For this review, take the finished solid that the model builds, in its own axes (mm). A direction names the side the tool comes from. Coordinates: 2 decimals unless noted, no trailing zeros. Loops run counter-clockwise (first coordinate to the right, second up) from the corner with the lowest first, then second, coordinate; pieces in that order, holes last. Notation, with made-up numbers: M -7,70.5 L 8,70.5 A28 cw 8,105.5 Z; hole C 26.25,64.25 d3. An arc over 180 degrees is marked long. Write item = value, one per line.
from build123d import *

# Parameters (mm, degrees)
SKETCH1_W           = 170
SKETCH1_H           = 130
BOSS_EXTRUDE1_DEPTH = 5
SKETCH2_W           = 67
SKETCH2_H           = 85
CUT_EXTRUDE1_DEPTH  = 108.121426428
SKETCH3_W           = 5
SKETCH3_H           = 5.833333
CUT_EXTRUDE2_DEPTH  = 108.121426428
FILLET1_R           = 15


with BuildPart() as part:
    # Sketch1 → Boss-Extrude1 (new body)
    with BuildSketch(Plane(origin=(0, 0, 0), x_dir=(1, 0, 0), z_dir=(0, 1, 0))):
        Rectangle(SKETCH1_W, SKETCH1_H)
    extrude(amount=BOSS_EXTRUDE1_DEPTH)

    # Sketch2 → Cut-Extrude1 (cut, through all)
    with BuildSketch(Plane(origin=(0, 5, 0), x_dir=(1, 0, 0), z_dir=(0, 1, 0))):
        Rectangle(SKETCH2_W, SKETCH2_H)
    extrude(amount=-CUT_EXTRUDE1_DEPTH, mode=Mode.SUBTRACT)

    # Sketch3 → Cut-Extrude2 (cut, through all)
    with BuildSketch(Plane(origin=(0, 5, 0), x_dir=(1, 0, 0), z_dir=(0, 1, 0))):
        with Locations((-36, -33.7500005)):
            Rectangle(SKETCH3_W, SKETCH3_H)
        with Locations((36, 33.7500005)):
            Rectangle(SKETCH3_W, SKETCH3_H)
        with Locations((-36, 33.7500005)):
            Rectangle(SKETCH3_W, SKETCH3_H)
        with Locations((36, -33.7500005)):
            Rectangle(SKETCH3_W, SKETCH3_H)
    extrude(amount=-CUT_EXTRUDE2_DEPTH, mode=Mode.SUBTRACT)

    # Fillet1
    fillet1_edges = [part.edges().sort_by_distance(p)[0] for p in [
        (85, 2.5, 65),
        (-85, 2.5, 65),
        (-85, 2.5, -65),
        (85, 2.5, -65),
    ]]
    fillet(fillet1_edges, radius=FILLET1_R)


solid = part.part
Q1. Machinability: for faces 1 (the face through (33.5, 3, -40)), 2 (the face through (80.49, 2.54, -60.72)), which of the approach directions +Z, -Z, +X, -X, +Y, -Y give a long, thin tool a straight path to every point of the face, cutting with its end or side? Answer none if there is none.
Solved:
face_1 = +Y, -Y
face_2 = -Z, +X, +Y, -Y
Q2. For line 1 along Z through (x, y) = (-35, 1.8); line 2 along X through (y, z) = (1.4, -26.5); line 3 along Z through (x, y) = (8, 2.95), list the stretches that pass through material, from the lowest coordinate up.
Solved:
line_1 = -65 to -36.67, -30.83 to 30.83, 36.67 to 65
line_2 = -85 to -33.5, 33.5 to 85
line_3 = -65 to -42.5, 42.5 to 65
Q3. Add section A-A (x = -17). Write out the cut boundary in (y, z), and give its area (3 significant figures).
Solved:
outline = M 0,-65 L 5,-65 L 5,-42.5 L 0,-42.5 Z; M 0,42.5 L 5,42.5 L 5,65 L 0,65 Z
area = 225 mm²
Q4. Add section B-B (y = 1.2). Write out the cut boundary in (x, z).
Solved:
outline = M -85,-50 A15 ccw -70,-65 L 70,-65 A15 ccw 85,-50 L 85,50 A15 ccw 70,65 L -70,65 A15 ccw -85,50 Z; hole M -38.5,-36.67 L -33.5,-36.67 L -33.5,-42.5 L 33.5,-42.5 L 33.5,-36.67 L 38.5,-36.67 L 38.5,-30.83 L 33.5,-30.83 L 33.5,30.83 L 38.5,30.83 L 38.5,36.67 L 33.5,36.67 L 33.5,42.5 L -33.5,42.5 L -33.5,36.67 L -38.5,36.67 L -38.5,30.83 L -33.5,30.83 L -33.5,-30.83 L -38.5,-30.83 Z
Q5. Draft analysis for pull direction X (two halves, no side actions). For faces 3 (the face through (-36, 3, 30.833)), 4 (the face through (-38.5, 3, 34)), 5 (the face through (80.49, 2.54, 60.72)), 6 (the face through (-80.72, 2.54, 60.49)), state which applies: +X half, -X half, draft (parallel to the pull), parting line (faces both ways), or undercut.
Solved:
face_3 = undercut
face_4 = undercut
face_5 = +X half
face_6 = -X half
